```python
from build123d import *

# Parameters (mm, degrees)
F0_R     = 24.13
F1_DEPTH = 330.2
F2_R     = 24.13
F3_R     = 24.13
F4_R     = 24.13
F5_DEPTH = 24.13


with BuildPart() as f1:
    # F0 (on Top) → F1 (new body)
    with BuildSketch(Plane.XY):
        Circle(F0_R)
    extrude(amount=F1_DEPTH)

    # F2
    f2_edges = [f1.edges().sort_by_distance(p)[0] for p in [
        (-24.13, 0, 330.2),
    ]]
    fillet(f2_edges, radius=F2_R)

    # F3
    f3_edges = [f1.edges().sort_by_distance(p)[0] for p in [
        (-24.13, 0, 0),
    ]]
    fillet(f3_edges, radius=F3_R)

    # F4 (on Front) → F5 (join)
    with BuildSketch(Plane.XZ):
        with Locations((0, 165.1)):
            Circle(F4_R)
    extrude(amount=F5_DEPTH)


solid = f1.part
```
Geometry check sheet. Reference: the model listing, model coordinates, mm. A direction names the side the tool comes from. Coordinates: 2 decimals unless noted, no trailing zeros. Write each loop counter-clockwise with the first axis right and the second up, starting at its lowest first coordinate (ties: lowest second). Pieces come first, ordered by that corner, then holes. Notation, with made-up numbers: M 36,-11.75 L 67,-11.75 A18 cw 67,9.25 Z; hole C 20.25,60.5 d4. An arc over 180 degrees is marked long. Use one line per item in the form item = value. Start each with the question number.
1) Section check B-B on x = 19. Enter the section's corners in (y, z).
2) Section check D-D on y = 10. Enter the section's corners in (x, z), and give its area (3 significant figures).
3) Section check C-C on z = 283. Enter the section's corners in (x, y).
4) Go/stop test with flat-tipped pins: pin 1 Ø3 at (y, z) = (-8, 192.5) entering from -X; pin 2 Ø10 at (y, z) = (-18, 94) entering from -X; pin 3 Ø4 at (x, z) = (-11.5, 234) entering from -Y. Record where each tip stops, or that it passes through.
5) Set-up check for faces 1 (the cylindrical face through (-24.13, -15.58, 165.28)), 2 (the flat face through (0, -24.13, 165)), 3 (the cylindrical face through (24.13, -15.58, 164.92)), 4 (the cylindrical face through (-3.141, 23.925, 163.126)): record each of +Z, -Z, +X, -X, +Y, -Y from which the full face is reachable in a straight line by a thin tool's end or side.
6) Thickness scan on probe 1 along Y at (x, z) = (-1, 138); probe 2 along Z at (x, y) = (7.5, 8); probe 3 along Z at (x, y) = (12.5, 18). Record the ranges inside material, lowest first. Write a range as from..to.
7) Section check A-A on y = -10. Enter the section's corners in (x, z), and give its area (3 significant figures).
Responses:
q1.outline = M -24.13,150.23 L -14.87,150.23 L -14.87,24.13 A14.87 ccw 14.87,24.13 L 14.87,306.07 A14.87 ccw -14.87,306.07 L -14.87,179.97 L -24.13,179.97 Z
q2.outline = M -21.96,24.13 A21.96 ccw 21.96,24.13 L 21.96,306.07 A21.96 ccw -21.96,306.07 Z
q2.area = 13,900 mm2
q3.outline = C 0,0 d48.26
q4.pin_1 = -23.24
q4.pin_2 = -20.33
q4.pin_3 = -22.18
q5.face_1 = -X, -Y
q5.face_2 = +Z, -Z, +X, -X, -Y
q5.face_3 = +X, -Y
q5.face_4 = none
q6.probe_1 = -24.11..24.11
q6.probe_2 = 2.64..327.56
q6.probe_3 = 14.03..316.17
q7.outline = M -21.96,24.13 A21.96 ccw 21.96,24.13 L 21.96,155.1 A24.13 ccw 21.96,175.1 L 21.96,306.07 A21.96 ccw -21.96,306.07 L -21.96,175.1 A24.13 ccw -21.96,155.1 Z
q7.area = 14,000 mm2
